from build123d import *

# Parameters (mm, degrees)
SKETCH117_R           = 3
CUT_EXTRUDE4_DEPTH    = 3
SKETCH122_R           = 6.539767279
BOSS_EXTRUDE1_DEPTH   = 5
SKETCH123_R           = 3.0360463
CUT_EXTRUDE5_DEPTH    = 5
M2X0_4_TAPPED_HOLE1_D = 1.6


with BuildPart() as part:
    # Sketch9 → Revolve1 (revolve)
    with BuildSketch(Plane.XY):
        with BuildLine():
            Line((-4.703089141, -2.935363462), (8.296910859, -2.935363462))
            Line((8.296910859, -2.935363462), (8.296910859, 0.064636538))
            Line((8.296910859, 0.064636538), (-4.703089141, 0.064636538))
            add(Edge.make_bspline(
                [(-4.703089141, 0.064636538), (0.132127885, -1.294166307), (-4.703089141, -2.935363462)],
                knots=[0, 0, 0, 1, 1, 1], degree=2))
        make_face()
    revolve(axis=Axis((8.296910859, -2.935363462, 0), (0, 1, 0)))

    # Sketch117 → Cut-Extrude4 (cut)
    with BuildSketch(Plane(origin=(0, 0.064636538, 0), x_dir=(1, 0, 0), z_dir=(0, 1, 0))):
        with Locations((8.29691086, 0)):
            Circle(SKETCH117_R)
    extrude(amount=-CUT_EXTRUDE4_DEPTH, mode=Mode.SUBTRACT)

    # Sketch122 → Boss-Extrude1 (add)
    with BuildSketch(Plane(origin=(0, -2.935363462, 0), x_dir=(-1, 0, 0), z_dir=(0, -1, 0))):
        with Locations((-8.29691086, 0)):
            Circle(SKETCH122_R)
    extrude(amount=BOSS_EXTRUDE1_DEPTH)

    # Sketch123 → Cut-Extrude5 (cut)
    with BuildSketch(Plane(origin=(0, -2.935363462, 0), x_dir=(1, 0, 0), z_dir=(0, 1, 0))):
        with Locations((8.33295716, 0)):
            Circle(SKETCH123_R)
    extrude(amount=-CUT_EXTRUDE5_DEPTH, mode=Mode.SUBTRACT)

    # M2x0.4 Tapped Hole1 (through all)
    with Locations(Plane(origin=(1.815385484, -5.431649491, -0.870852953), x_dir=(0.133162682, 0, -0.991094193), z_dir=(-0.991094193, 0, -0.133162682))):
        with Locations((0, 0)):
            Hole(M2X0_4_TAPPED_HOLE1_D / 2)


solid = part.part
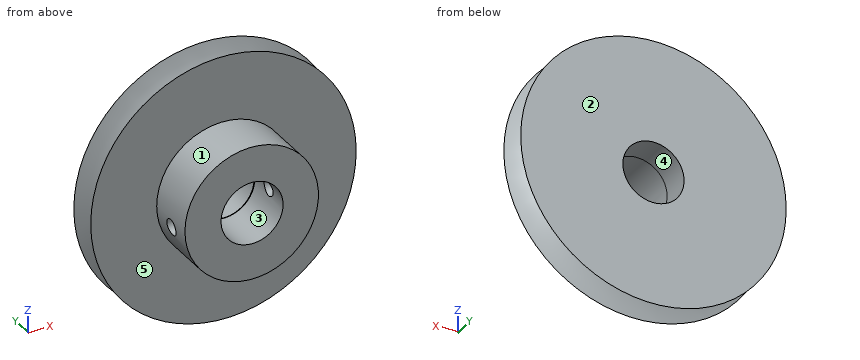
Input: part model. Units: mm. Frame: model coordinates. Face numbers are marked on the shaded views. A direction names the side the tool comes from. Give positions to 0.01 mm unless a question says otherwise; leave off trailing zeros. Write each loop counter-clockwise with the first axis right and the second up, starting at its lowest first coordinate (ties: lowest second). Pieces come first, ordered by that corner, then holes. Notation, with made-up numbers: M 62,3.25 L 72,3.25 A26 cw 72,41.25 Z; hole C -36,-13.75 d2. An arc over 180 degrees is marked long. Use one line per item in the form item = value.
1. Cut plane A-A on y = -7.25. Return loops of the section in (x, z).
Outcome:
outline = C 8.3,0 d13.08; hole C 8.33,0 d6.07
2. Reachability of the marked faces 4 and 5 from +Z, -Z, +X, -X, +Y, -Y: full face, straight path, thin tool, end or side. Return the list, or none.
Outcome:
face_4 = +Y, -Y
face_5 = -Y
3. Mould query, pull axis Z, two halves, no side actions, for the marked faces 1, 2 and 3. Classes: released by +Z, released by -Z, zero draft, split by the parting line, or undercut.
Outcome:
face_1 = split by the parting line
face_2 = zero draft
face_3 = undercut
4. Ray query, L1, parallel to Z at x = 8.25, y = -3.25; L2, parallel to X at y = -4.6, z = 0; L3, parallel to Y at x = -0.5, z = -8.5. Return the intervals inside material, ascending.
Outcome:
L1 = -6.54 to -3.03, 3.03 to 6.54
L2 = 1.76 to 5.3, 11.37 to 14.84
L3 = -2.94 to -2.65, -0.17 to 0.06
